```python
from build123d import *

# Parameters (mm, degrees)
ESQUISSE1_R             = 10
BOSS_EXTRU_1_DEPTH      = 20
ESQUISSE2_W             = 128.799029074
ESQUISSE2_H             = 20
ESQUISSE2_W_2           = 74.303027804
BOSS_EXTRU_2_DEPTH      = 20
ESQUISSE3_R             = 10
BOSS_EXTRU_3_DEPTH      = 20
CHANFREIN3_SIZE         = 10
ESQUISSE2_5_W           = 74.303027804
ESQUISSE2_5_H           = 20
BOSS_EXTRU_4_DEPTH      = 60
ESQUISSE4_R             = 10
ENL_V_MAT_EXTRU_1_DEPTH = 831.815461604
CHANFREIN2_SIZE         = 10


with BuildPart() as part:
    # Esquisse1 → Boss.-Extru.1 (new body)
    with BuildSketch(Plane.XY):
        Polygon((455.162466111, 170), (485.162466111, 170), (535.244755063, -80), (406.445725989, -80), align=None)
        with Locations(Location((470.845240526, 150, 0), (0, 0, 180))):
            Circle(ESQUISSE1_R, mode=Mode.SUBTRACT)
    extrude(amount=BOSS_EXTRU_1_DEPTH)

    # Esquisse2 → Boss.-Extru.2 (add)
    with BuildSketch(Plane.XZ.offset(80)):
        Polygon((735.244755063, -25), (735.244755063, 20), (535.244755063, 20), (535.244755063, 0), (406.445725989, 0), (406.445725989, -25), align=None)
        with Locations((470.845240526, 10)):
            Rectangle(ESQUISSE2_W, ESQUISSE2_H)
        Polygon((735.244755063, -70), (735.244755063, -25), (406.445725989, -25), (406.445725989, -50), (535.244755063, -50), (535.244755063, -70), align=None)
        Polygon((331.553149283, 20), (406.445725989, 20), (-22.137924362, 277.519037455), (-42.004245202, 244.455927292), align=None)
        Polygon((406.445725989, 0), (406.445725989, 20), (331.553149283, 20), (406.445725989, -25), align=None)
        Polygon((256.445725989, -25), (406.445725989, -25), (331.553149283, 20), (330.748753793, 20), (330.748753793, 0), (256.445725989, 0), align=None)
        Polygon((331.553149283, -70), (406.445725989, -25), (256.445725989, -25), (256.445725989, -50), (330.748753793, -50), (330.748753793, -70), align=None)
        Polygon((406.445725989, -50), (406.445725989, -25), (331.553149283, -70), (406.445725989, -70), align=None)
        with Locations((470.845240526, -60)):
            Rectangle(ESQUISSE2_W, ESQUISSE2_H)
        Polygon((406.445725989, -70), (331.553149283, -70), (-42.004245202, -294.455927292), (-22.137924362, -327.519037455), align=None)
        with Locations((293.597239891, 10)):
            Rectangle(ESQUISSE2_W_2, ESQUISSE2_H)
        with Locations((293.597239891, -60)):
            Rectangle(ESQUISSE2_W_2, ESQUISSE2_H)
    extrude(amount=BOSS_EXTRU_2_DEPTH)

    # Esquisse3 → Boss.-Extru.3 (add)
    with BuildSketch(Plane(origin=(0, 0, -70), x_dir=(-1, 0, 0), z_dir=(0, 0, -1))):
        Polygon((-406.445725989, -80), (-455.162466111, 170), (-485.162466111, 170), (-535.244755063, -80), align=None)
        with Locations((-470.845240526, 150)):
            Circle(ESQUISSE3_R, mode=Mode.SUBTRACT)
    extrude(amount=-BOSS_EXTRU_3_DEPTH)

    # Chanfrein3
    chanfrein3_edges = [part.edges().sort_by_distance(p)[0] for p in [
        (192.153900813, -80, 148.759518728),
        (144.774452041, -80, -182.227963646),
        (192.153900813, -80, -198.759518728),
        (144.774452041, -80, 132.227963646),
    ]]
    chamfer(chanfrein3_edges, length=CHANFREIN3_SIZE)

    # Esquisse2_5 → Boss.-Extru.4 (add)
    with BuildSketch(Plane.XZ.offset(80)):
        with Locations((293.597239891, -60)):
            Rectangle(ESQUISSE2_5_W, ESQUISSE2_5_H)
        with Locations((293.597239891, 10)):
            Rectangle(ESQUISSE2_5_W, ESQUISSE2_5_H)
    extrude(amount=-BOSS_EXTRU_4_DEPTH)

    # Esquisse4 → Enl_v. mat.-Extru.1 (cut, through all)
    with BuildSketch(Plane(origin=(0, 0, -70), x_dir=(-1, 0, 0), z_dir=(0, 0, -1))):
        with Locations((-293.597239891, -40)):
            Circle(ESQUISSE4_R)
    extrude(amount=-ENL_V_MAT_EXTRU_1_DEPTH, mode=Mode.SUBTRACT)

    # Chanfrein2
    chanfrein2_edges = [part.edges().sort_by_distance(p)[0] for p in [
        (635.244755063, -80, 20),
        (735.244755063, -80, -25),
        (635.244755063, -80, -70),
    ]]
    chamfer(chanfrein2_edges, length=CHANFREIN2_SIZE)


solid = part.part
```
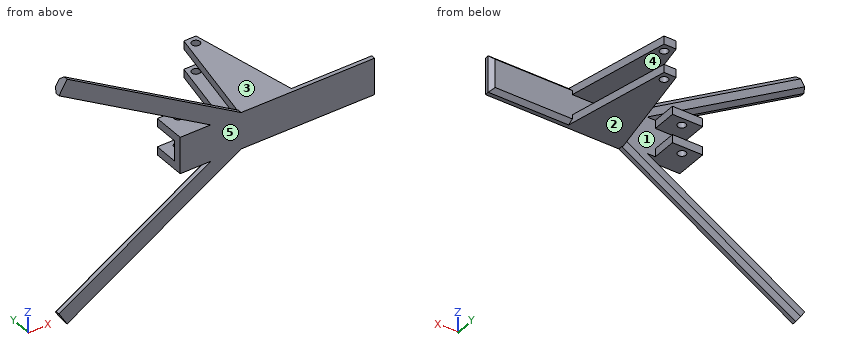
Build history of the part. All positions in model axes, mm. Face numbers are marked on the shaded views. A direction names the side the tool comes from. Coordinates: 2 decimals unless noted, no trailing zeros. Order: outer loops, then holes, each group sorted by start corner. A loop starts at its lowest first (then second) coordinate and runs counter-clockwise, first axis right, second up. Notation, with made-up numbers: (61.5, 1) -> (119.5, 1) arc R25 ccw to (119.5, 18) -> close; hole circle Ø5 at (46.5, 76.25). An arc over 180 degrees is marked (long way). Answer in a Markdown table with one row per item. Add a question column.
Q1. Which spindle directions (+Z, -Z, +X, -X, +Y, -Y) get a long thin tool onto all of the face, cutting with end or side? Do the marked faces 4 and 5. Say none if no direction does.
Q2. Band-saw the part on A-A, the plane y = -40. List the corners of the cut face in (x, z).
Q3. Drop flat-ended pins along their axis: pin 1 (22 mm diameter, centred on y = -40.5, z = -61, fed in from +X); pin 2 (23 mm diameter, centred on x = 293.6, y = -40, fed in from -Z); pin 3 (18 mm diameter, centred on x = 293.6, y = -40, fed in from -Z); pin 4 (16 mm diameter, centred on x = 283.5, z = -60, fed in from +Y). Give the stop position or say it passes through.
Q4. Mould opens along Z. For the marked faces 1, 2 and 3 say: +Z half, -Z half, draft (parallel to the pull), parting line (faces both ways), or undercut.
Q5. Band-saw the part on D-D, the plane y = 41.5. List the corners of the cut face in (x, z), then the cut area to 3 significant figures.
Q6. Band-saw the part on B-B, the plane z = -29.5. List the corners of the cut face in (x, y).
Q7. Wall check: line 1 along Z through (x, y) = (438.5, -19); line 2 along Y through (x, z) = (355, -28); line 3 along X through (y, z) = (-62, -69). Give the ranges that are in metal, low to high. Write a range as [from, to].
Q8. Band-saw the part on C-C, the plane x = 100.5. List the corners of the cut face in (y, z), then the cut area to 3 significant figures.
Answers follow:
| question | item | result |
|---|---|---|
| 1 | face 4 | +X, -X, +Y |
| 1 | face 5 | +Z, -Z, +X, -X, -Y |
| 2 | outline | (256.45, -70) -> (283.6, -70) -> (283.6, -50) -> (256.45, -50) -> close; (256.45, 0) -> (283.6, 0) -> (283.6, 20) -> (256.45, 20) -> close; (303.6, -70) -> (330.75, -70) -> (330.75, -50) -> (303.6, -50) -> close; (303.6, 0) -> (330.75, 0) -> (330.75, 20) -> (303.6, 20) -> close; (414.24, -70) -> (527.23, -70) -> (527.23, -50) -> (414.24, -50) -> close; (414.24, 0) -> (527.23, 0) -> (527.23, 20) -> (414.24, 20) -> close |
| 3 | pin 1 | x = 529.54 |
| 3 | pin 2 | z = -70 |
| 3 | pin 3 | through |
| 3 | pin 4 | y = -20 |
| 4 | face 1 | undercut |
| 4 | face 2 | -Z half |
| 4 | face 3 | +Z half |
| 5 | outline | (430.12, -70) -> (510.9, -70) -> (510.9, -50) -> (430.12, -50) -> close; (430.12, 0) -> (510.9, 0) -> (510.9, 20) -> (430.12, 20) -> close |
| 5 | area | 3,230 mm^2 |
| 6 | outline | (256.45, -100) -> (735.24, -100) -> (735.24, -90) -> (725.24, -80) -> (256.45, -80) -> close |
| 7 | line 1 | [-70, -50], [0, 20] |
| 7 | line 2 | [-100, -80] |
| 7 | line 3 | [256.45, 330.75], [409.95, 531.64] |
| 8 | outline | (-100, -253.83) -> (-90, -253.83) -> (-80, -242.16) -> (-80, -220.5) -> (-90, -208.83) -> (-100, -208.83) -> close; (-100, 158.83) -> (-90, 158.83) -> (-80, 170.5) -> (-80, 192.16) -> (-90, 203.83) -> (-100, 203.83) -> close |
| 8 | area | 1,570 mm^2 |
